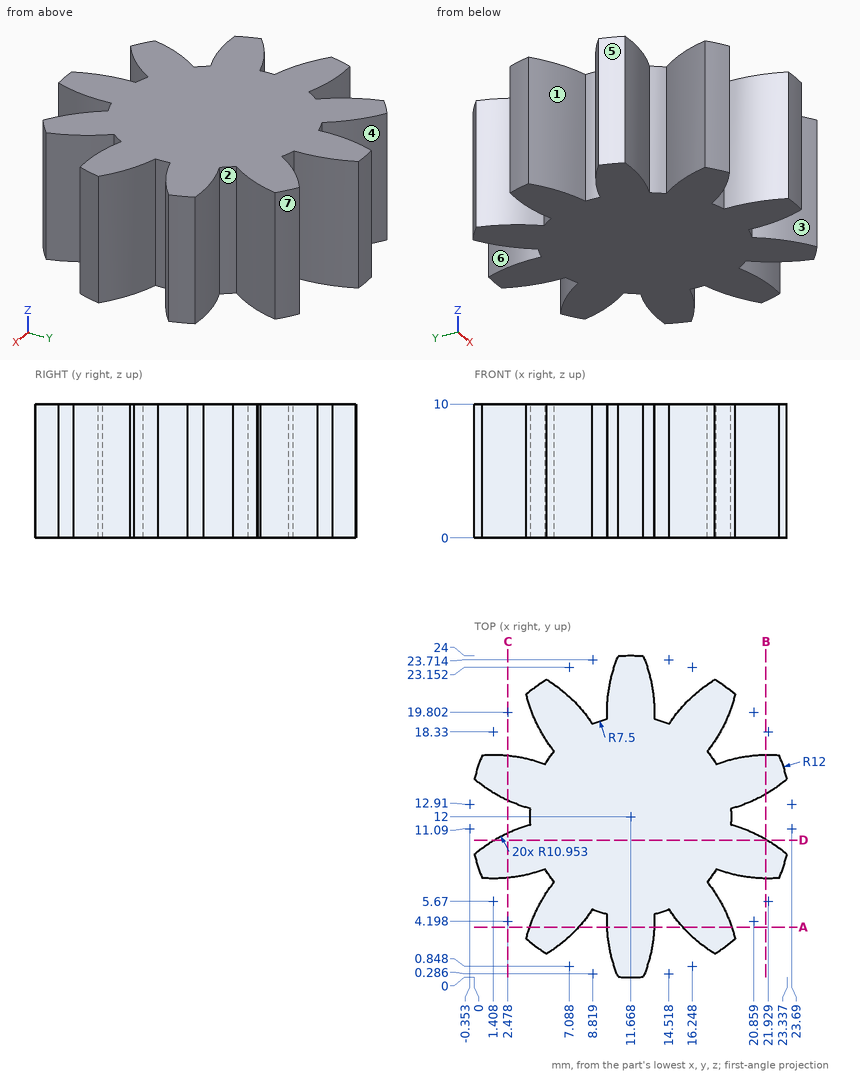
Geometry check sheet. Reference: drawing and pictorial views, mm from the part's lowest x, y, z. A direction names the side the tool comes from. Give positions to 0.01 mm unless a question says otherwise; leave off trailing zeros. Write each loop counter-clockwise with the first axis right and the second up, starting at its lowest first coordinate (ties: lowest second). Pieces come first, ordered by that corner, then holes.
Item 1: Cross-section at D-D (y = 10.25). Enter the section's corners in (x, z).
Item 2: Cross-section at A-A (y = 3.75). Enter the section's corners in (x, z) (1 decimal), and give its area (3 significant figures).
Item 3: Access from +Z, -Z, +X, -X, +Y, -Y to the whole of each face (thin tool, end or side, straight path). Record for the marked faces 1, 2, 3 and 4.
Item 4: Gauge pin test, flat ends, axial feed: pin 1 (1 mm diameter, centred on y = 12, z = 1.5, fed in from -X); pin 2 (1 mm diameter, centred on x = 6, z = 3.5, fed in from -Y); pin 3 (3 mm diameter, centred on y = 17.5, z = 2.5, fed in from +X). Record the tip position at first contact, or that the pin passes through.
Item 5: Cross-section at B-B (x = 21.75). Enter the section's corners in (y, z).
Item 6: Scan lines: L1, parallel to X at y = 20.25, z = 5.25 (1 decimal); L2, parallel to X at y = 4, z = 6.5 (1 decimal); L3, parallel to Y at x = 18.25, z = 7 (1 decimal). Record each from-to range of solid material in increasing order.
Item 7: Cross-section at C-C (x = 2.5). Enter the section's corners in (y, z) (1 decimal).
Item 8: Draft check along X on the marked faces 5, 6 and 7. Enter one of: released by +X, released by -X, zero draft, split by the parting line, or undercut.
Report:
1. outline: (1.47, 0) - (21.87, 0) - (21.87, 10) - (1.47, 10) - close
2. outline: (4.1, 0) - (7.8, 0) - (7.8, 10) - (4.1, 10) - close; (9.9, 0) - (13.4, 0) - (13.4, 10) - (9.9, 10) - close; (15.6, 0) - (19.2, 0) - (19.2, 10) - (15.6, 10) - close
2. area: 108 mm2
3. face 1: +Z, -Z, -X
3. face 2: +Z, -Z
3. face 3: +Z, -Z, -Y
3. face 4: +Z, -Z, +Y
4. pin 1: stops at x = 4.17
4. pin 2: stops at y = 1.83
4. pin 3: stops at x = 22.98
5. outline: (7.38, 0) - (10.32, 0) - (10.32, 10) - (7.38, 10) - close; (13.68, 0) - (16.62, 0) - (16.62, 10) - (13.68, 10) - close
6. L1: x = 4.1 to 7.8, 9.9 to 13.4, 15.6 to 19.2
6. L2: x = 4.2 to 8, 9.9 to 13.4, 15.3 to 19.1
6. L3: y = 2 to 5.9, 8 to 16, 18.1 to 22
7. outline: (7.4, 0) - (10.8, 0) - (10.8, 10) - (7.4, 10) - close; (13.2, 0) - (16.6, 0) - (16.6, 10) - (13.2, 10) - close
8. face 5: released by -X
8. face 6: undercut
8. face 7: released by +X
